```python
from build123d import *

# Parameters (mm, degrees)
BOSS_EXTRUDE1_DEPTH = 10.9032
SKETCH2_W           = 9
SKETCH2_H           = 0.5
CUT_EXTRUDE1_DEPTH  = 13.01999980199667
FILLET1_R           = 0.2
SWEEP1_START        = -3.3
SWEEP1_DEPTH        = 3.05
SWEEP1_2_ANGLE      = 90
FILLET2_R           = 0.5


with BuildPart() as part:
    # Sketch1 → Boss-Extrude1 (new body)
    with BuildSketch(Plane.XY):
        with BuildLine():
            Line((-4.225, 0.7750000000000001), (4.225, 0.7750000000000001))
            ThreePointArc((4.225, 0.7750000000000001), (5, 0), (4.225, -0.7750000000000001))
            Line((4.225, -0.7750000000000001), (-4.225, -0.7750000000000001))
            ThreePointArc((-4.225, -0.7750000000000001), (-5, 9e-17), (-4.225, 0.7750000000000001))
        make_face()
    extrude(amount=BOSS_EXTRUDE1_DEPTH)

    # Sketch2 → Cut-Extrude1 (cut, through all)
    with BuildSketch(Plane.XY.offset(10.9032)):
        Rectangle(SKETCH2_W, SKETCH2_H)
    extrude(amount=-CUT_EXTRUDE1_DEPTH, mode=Mode.SUBTRACT)

    # Fillet1
    fillet1_edges = [part.edges().sort_by_distance(p)[0] for p in [
        (4.500000000000003, 0.2500000000000001, 5.4516),
        (4.500000000000003, -0.2499999999999999, 5.4516),
        (-4.499999999999997, -0.2499999999999999, 5.4516),
        (-4.499999999999997, 0.2500000000000001, 5.4516),
    ]]
    fillet(fillet1_edges, radius=FILLET1_R)

    # Sweep1: read off the stored shape, not the designer's step
    # Sweep1 outline → Sweep1 (add)
    with BuildSketch(Plane(origin=(0, 0, 0), x_dir=(1, 0, 0), z_dir=(0, 1, 0)).offset(SWEEP1_START)):
        with BuildLine():
            Line((-4.225, -11.9782), (4.225, -11.9782))
            ThreePointArc((4.225, -11.9782), (5, -11.2032), (4.225, -10.4282))
            Line((4.225, -10.4282), (-4.225, -10.4282))
            ThreePointArc((-4.225, -10.4282), (-5, -11.2032), (-4.225, -11.9782))
        make_face()
    extrude(amount=SWEEP1_DEPTH)

    # Sweep1 2 outline → Sweep1 2 (revolve)
    with BuildSketch(Plane(origin=(0, -0.3, 10.9032), x_dir=(0, 1, -1.44e-15), z_dir=(0, -1.44e-15, -1))):
        with BuildLine():
            Line((0, 4.939580296), (0, -4.939580296))
            add(Edge.make_bspline(
                [(0, -4.939580296), (0.0519570394689895, -4.961393256983593), (0.10841554643003581, -4.979542137191699), (0.1692061790231751, -4.992872607462927), (0.23352242585972577, -5.000000001245932), (0.538087621369197, -4.999999995537749), (0.8228689184127496, -4.905109045106682), (1.0076156687544926, -4.675143876063141), (1.075000000000001, -4.4268164646885895), (1.075, -4.225)],
                knots=[1.5386603530075902, 1.5386603530075902, 1.5386603530075902, 1.5386603530075902, 1.5386603530075902, 1.5386603530075902, 1.968277128944731, 1.968277128944731, 1.968277128944731, 1.968277128944731, 3.5069374819523116, 3.5069374819523116, 3.5069374819523116, 3.5069374819523116, 3.5069374819523116, 3.5069374819523116], degree=5, weights=[1, 0.9999999999999993, 1.0001144222703127, 1.000064472262904, 1.0000000000000007, 1.0000000000000002, 0.9635119774531175, 0.9749056251717576, 1.000000000000001, 1]))
            Line((1.075, -4.225), (1.075, 4.225))
            add(Edge.make_bspline(
                [(1.075, 4.225), (1.0750000000000006, 4.426816468221435), (1.0076156662304492, 4.6751438856768095), (0.8228689080824526, 4.905109057133026), (0.5380876027644639, 5.000000001939648), (0.23352240972853552, 4.999999999458421), (0.16920616758934218, 4.992872604955472), (0.10841553935261468, 4.97954213491664), (0.05195703621157381, 4.961393255616055), (0, 4.939580296)],
                knots=[4.744524927237428, 4.744524927237428, 4.744524927237428, 4.744524927237428, 4.744524927237428, 4.744524927237428, 6.283185307179587, 6.283185307179587, 6.283185307179587, 6.283185307179587, 6.712802056182165, 6.712802056182165, 6.712802056182165, 6.712802056182165, 6.712802056182165, 6.712802056182165], degree=5, weights=[1, 0.9999999999999987, 0.9749056227861467, 0.9635119748925262, 1.0000000000000018, 1.0000000000000044, 1.0000644722550744, 1.0001144222464367, 0.999999999999996, 1]))
        make_face()
    revolve(axis=Axis((0, -0.3, 10.9032), (1, 0, 0)), revolution_arc=SWEEP1_2_ANGLE)

    # Fillet2
    fillet2_edges = [part.edges().sort_by_distance(p)[0] for p in [
        (-4.999999999999999, -3.3, 11.203199999999999),
        (0, -3.3, 10.4282),
        (4.999999999999999, -3.3, 11.203199999999999),
        (0, -3.3, 11.9782),
    ]]
    fillet(fillet2_edges, radius=FILLET2_R)


solid = part.part
```
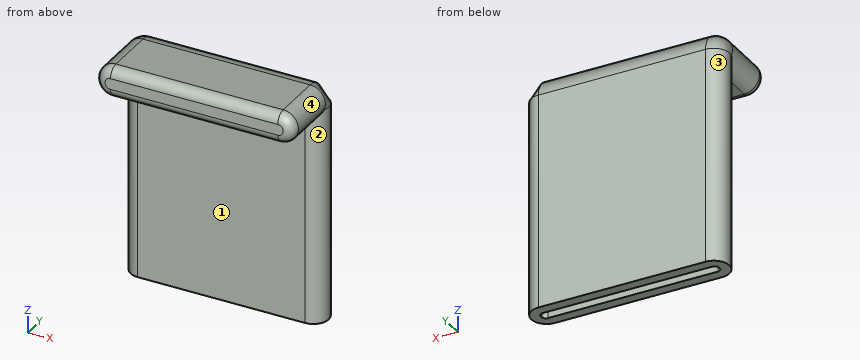
CAD build for the part. Positions are in the model's coordinates, mm. Face numbers are marked on the shaded views. A direction names the side the tool comes from. Coordinates: 2 decimals unless noted, no trailing zeros. Order: outer loops, then holes, each group sorted by start corner. A loop starts at its lowest first (then second) coordinate and runs counter-clockwise, first axis right, second up. Notation, with made-up numbers: (84.25, 65) - (89.25, 65) arc R31 cw to (89.25, 92) - close; hole circle Ø1 at (-38, 45). An arc over 180 degrees is marked (long way). Use a Markdown table: item, result. Add a question column.
(1) Flat gauge pins, fed straight in: pin 1 (1 mm diameter, centred on y = -1, z = 10.5, fed in from -X); pin 2 (0.6 mm diameter, centred on x = 1.5, y = -1.5, fed in from -Z). Where does each tip first touch, or does it go through?
(2) Drill centre lines: line 1 along Y through (x, z) = (-2, 3.25) (3 decimals); line 2 along X through (y, z) = (0, 4.5); line 3 along Z through (x, y) = (1.75, -1). Where is each one in solid material? Low to high. Write a range as [from, to].
(3) Saw through at C-C (y = -2.2). Give the cut face in (x, z) (3 decimals).
(4) Saw through at B-B (x = -1.5). Give the cut face in (y, z) (3 decimals).
(5) Which spindle directions (+Z, -Z, +X, -X, +Y, -Y) get a long thin tool onto all of the face, cutting with end or side? Do the marked faces 1, 2, 3 and 4. Say none if no direction does.
(6) Saw through at A-A (z = 3). Give the cut face in (x, y) (3 decimals), then the cut area to 3 significant figures.
Solved:
| question | item | result |
|---|---|---|
| 1 | pin 1 | stops at x = -4.97 |
| 1 | pin 2 | stops at z = 10.43 |
| 2 | line 1 | y = [-0.775, -0.25], [0.25, 0.775] |
| 2 | line 2 | x = [-5, -4.5], [4.5, 5] |
| 2 | line 3 | z = [10.43, 11.98] |
| 3 | outline | (-4.225, 10.428) - (4.225, 10.428) arc R0.775 ccw to (4.225, 11.978) - (-4.225, 11.978) arc R0.775 ccw to start |
| 4 | outline | (-3.3, 10.928) arc R0.5 ccw to (-2.8, 10.428) - (-0.775, 10.428) - (-0.775, 0) - (-0.25, 0) - (-0.25, 10.903) - (0.25, 10.903) - (0.25, 0) - (0.775, 0) - (0.775, 10.903) arc R1.075 ccw to (-0.3, 11.978) - (-2.8, 11.978) arc R0.5 ccw to (-3.3, 11.478) - close |
| 5 | face 1 | -Z, +X, -X, -Y |
| 5 | face 2 | -Z, +X |
| 5 | face 3 | -Z, -X |
| 5 | face 4 | +X, -Y |
| 6 | outline | (-4.225, -0.775) - (4.225, -0.775) arc R0.775 ccw to (4.225, 0.775) - (-4.225, 0.775) arc R0.775 ccw to start; hole (-4.5, -0.05) arc R0.2 ccw to (-4.3, -0.25) - (4.3, -0.25) arc R0.2 ccw to (4.5, -0.05) - (4.5, 0.05) arc R0.2 ccw to (4.3, 0.25) - (-4.3, 0.25) arc R0.2 ccw to (-4.5, 0.05) - close |
| 6 | area | 10.5 mm² |
